Design review of the part built by this model. Coordinates are the model's own, in mm. A direction names the side the tool comes from. Give positions to 0.01 mm unless a question says otherwise; leave off trailing zeros. Write each loop counter-clockwise with the first axis right and the second up, starting at its lowest first coordinate (ties: lowest second). Pieces come first, ordered by that corner, then holes. Notation, with made-up numbers: M 80,17.25 L 126,17.25 A7 cw 126,27.25 Z; hole C 81,53.25 d7. An arc over 180 degrees is marked long. Write each question's results on one line, items separated by ' | '. Start each with the question number.
from build123d import *

# Parameters (mm, degrees)
SKETCH1_W                = 40
SKETCH1_H                = 30
BOSS_EXTRUDE1_DEPTH      = 90
SHELL1_T                 = -4
FILLET1_R                = 5
CUT_EXTRUDE1_DEPTH       = 94.407708461
CUT_EXTRUDE1_DEPTH_BACK  = 94.407708461
CUT_EXTRUDE2_DEPTH       = 94.407708461
CUT_EXTRUDE2_DEPTH_BACK  = 94.407708461
SKETCH3_W                = 17.5
SKETCH3_H                = 40
SKETCH5_W                = 2
SKETCH5_H                = 40
BOSS_EXTRUDE2_DEPTH      = 3
SKETCH6_W                = 2
SKETCH6_H                = 18
BOSS_EXTRUDE3_DEPTH      = 3
SKETCH8_W                = 50
SKETCH8_H                = 50
BOSS_EXTRUDE4_DEPTH      = 18
SKETCH10_W               = 45
SKETCH10_H               = 10
CUT_EXTRUDE4_DEPTH       = 37.5
BOSS_EXTRUDE5_REACH      = 103.502
SKETCH15_W               = 10
SKETCH15_H               = 10
CUT_EXTRUDE8_DEPTH       = 103.988587343
CUT_EXTRUDE8_DEPTH_BACK  = 103.988587343
SKETCH20_R               = 2
SKETCH21_R               = 4
CUT_EXTRUDE9_DEPTH       = 5
SKETCH23_W               = 2
SKETCH23_H               = 15
CUT_EXTRUDE10_DEPTH      = 10
CUT_EXTRUDE11_START      = -10
SKETCH24_R               = 1.5
CUT_EXTRUDE11_DEPTH      = 116.031657717
CUT_EXTRUDE12_DEPTH      = 99.140965569
CUT_EXTRUDE12_DEPTH_BACK = 99.140965569
SKETCH27_W               = 50
SKETCH27_H               = 25
SKETCH29_W               = 50
SKETCH29_H               = 2
CUT_EXTRUDE13_DEPTH      = 2
SKETCH30_W               = 50
SKETCH30_H               = 2
CUT_EXTRUDE14_DEPTH      = 2
CUT_EXTRUDE15_DEPTH      = 99.140965569
CUT_EXTRUDE15_DEPTH_BACK = 99.140965569
SKETCH31_R               = 2
SKETCH33_R               = 4
CUT_EXTRUDE16_DEPTH      = 15


with BuildPart() as part:
    # Sketch1 → Boss-Extrude1 (new body)
    with BuildSketch(Plane(origin=(0, 0, 0), x_dir=(1, 0, 0), z_dir=(0, 1, 0))):
        Rectangle(SKETCH1_W, SKETCH1_H)
    extrude(amount=BOSS_EXTRUDE1_DEPTH)

    # Shell1
    shell1_openings = [part.faces().sort_by_distance(p)[0] for p in [
        (0, 90, 0),
        (0, 0, 0),
    ]]
    offset(amount=SHELL1_T, openings=shell1_openings, kind=Kind.INTERSECTION)

    # Fillet1
    fillet1_edges = [part.edges().sort_by_distance(p)[0] for p in [
        (20, 45, 15),
        (-20, 45, 15),
        (-20, 45, -15),
        (20, 45, -15),
    ]]
    fillet(fillet1_edges, radius=FILLET1_R)

    # Sketch2 → Cut-Extrude1 (cut, two sides: drawn at the far end of the back side and taken through both)
    with BuildSketch(Plane.XY.offset(-CUT_EXTRUDE1_DEPTH_BACK)):
        Polygon((-5.5, 90), (-20, 66), (-20, 90), align=None)
    extrude(amount=CUT_EXTRUDE1_DEPTH + CUT_EXTRUDE1_DEPTH_BACK, mode=Mode.SUBTRACT)

    # Sketch3 → Cut-Extrude2 (cut, two sides: drawn at the far end of the back side and taken through both)
    with BuildSketch(Plane.XY.offset(-CUT_EXTRUDE2_DEPTH_BACK)):
        with Locations((11.25, 70)):
            Rectangle(SKETCH3_W, SKETCH3_H)
    extrude(amount=CUT_EXTRUDE2_DEPTH + CUT_EXTRUDE2_DEPTH_BACK, mode=Mode.SUBTRACT)

    # Sketch5 → Boss-Extrude2 (add)
    with BuildSketch(Plane(origin=(2.5, 0, 0), x_dir=(0, 0, -1), z_dir=(1, 0, 0))):
        with Locations((-13, 70)):
            Rectangle(SKETCH5_W, SKETCH5_H)
    boss_extrude2 = extrude(amount=BOSS_EXTRUDE2_DEPTH)

    # Mirror1: Boss-Extrude2 across plane
    add(boss_extrude2.mirror(Plane.XY))

    # Sketch6 → Boss-Extrude3 (add)
    with BuildSketch(Plane(origin=(-43.86391097, 26.501112878, 0), x_dir=(0, 0, 1), z_dir=(-0.8559155419457906, 0.5171156399255814, 0))):
        with Locations((-13, 65.188262756)):
            Rectangle(SKETCH6_W, SKETCH6_H)
    boss_extrude3 = extrude(amount=BOSS_EXTRUDE3_DEPTH)

    # Mirror2: Boss-Extrude3 across plane
    add(boss_extrude3.mirror(Plane.XY))

    # Sketch8 → Boss-Extrude4 (add)
    with BuildSketch(Plane(origin=(0, 0, 0), x_dir=(1, 0, 0), z_dir=(0, 1, 0))):
        Rectangle(SKETCH8_W, SKETCH8_H)
    extrude(amount=-BOSS_EXTRUDE4_DEPTH)

    # Sketch10 → Cut-Extrude4 (cut)
    with BuildSketch(Plane.ZY.offset(25)):
        with Locations((0, -9)):
            Rectangle(SKETCH10_W, SKETCH10_H)
    extrude(amount=-CUT_EXTRUDE4_DEPTH, mode=Mode.SUBTRACT)

    # Sketch15 → Boss-Extrude5 (add, up to next)
    with BuildSketch(Plane.XY.offset(-11), mode=Mode.PRIVATE) as boss_extrude5_sk1:
        with Locations((-11, 5)):
            Rectangle(SKETCH15_W, SKETCH15_H)
    boss_extrude5_tool1 = extrude(boss_extrude5_sk1.sketch, amount=BOSS_EXTRUDE5_REACH, mode=Mode.PRIVATE) - part.part
    add(boss_extrude5_tool1.solids().sort_by_distance((-11, 5, -11))[0])

    # Sketch20 → Cut-Extrude8 (cut, two sides: drawn at the far end of the back side and taken through both)
    with BuildSketch(Plane(origin=(0, 0, -15), x_dir=(-1, 0, 0), z_dir=(0, 0, -1)).offset(-CUT_EXTRUDE8_DEPTH_BACK)):
        with Locations((11, 5)):
            Circle(SKETCH20_R)
    extrude(amount=CUT_EXTRUDE8_DEPTH + CUT_EXTRUDE8_DEPTH_BACK, mode=Mode.SUBTRACT)

    # Sketch21 → Cut-Extrude9 (cut)
    with BuildSketch(Plane(origin=(0, 0, -15), x_dir=(-1, 0, 0), z_dir=(0, 0, -1))):
        with Locations((11, 5)):
            Circle(SKETCH21_R)
    cut_extrude9 = extrude(amount=-CUT_EXTRUDE9_DEPTH, mode=Mode.SUBTRACT)

    # Mirror3: Cut-Extrude9 across plane
    add(cut_extrude9.mirror(Plane.XY), mode=Mode.SUBTRACT)

    # Sketch23 → Cut-Extrude10 (cut)
    with BuildSketch(Plane(origin=(0, 50, 0), x_dir=(1, 0, 0), z_dir=(0, 1, 0))):
        with Locations((17.949489743, 0)):
            Rectangle(SKETCH23_W, SKETCH23_H)
    extrude(amount=-CUT_EXTRUDE10_DEPTH, mode=Mode.SUBTRACT)

    # Sketch24 → Cut-Extrude11 (cut)
    with BuildSketch(Plane(origin=(20, 0, 0), x_dir=(0, 0, -1), z_dir=(1, 0, 0)).offset(CUT_EXTRUDE11_START)):
        with Locations(Location((-5, 46, 0), (0, 0, 180))):
            Circle(SKETCH24_R)
    cut_extrude11 = extrude(amount=CUT_EXTRUDE11_DEPTH, mode=Mode.SUBTRACT)

    # Mirror4: Cut-Extrude11 across plane
    add(cut_extrude11.mirror(Plane.XY), mode=Mode.SUBTRACT)

    # Sketch27 → Cut-Extrude12 (cut, two sides: drawn at the far end of the back side and taken through both)
    with BuildSketch(Plane(origin=(0, 0, 0), x_dir=(1, 0, 0), z_dir=(0, 1, 0)).offset(-CUT_EXTRUDE12_DEPTH_BACK)):
        with Locations((0, -12.5)):
            Rectangle(SKETCH27_W, SKETCH27_H)
    extrude(amount=CUT_EXTRUDE12_DEPTH + CUT_EXTRUDE12_DEPTH_BACK, mode=Mode.SUBTRACT)

    # Sketch29 → Cut-Extrude13 (cut)
    with BuildSketch(Plane.XY):
        with Locations((0, -2)):
            Rectangle(SKETCH29_W, SKETCH29_H)
    extrude(amount=-CUT_EXTRUDE13_DEPTH, mode=Mode.SUBTRACT)

    # Sketch30 → Cut-Extrude14 (cut)
    with BuildSketch(Plane.XY):
        with Locations((0, -16)):
            Rectangle(SKETCH30_W, SKETCH30_H)
    extrude(amount=-CUT_EXTRUDE14_DEPTH, mode=Mode.SUBTRACT)

    # Sketch31 → Cut-Extrude15 (cut, two sides: drawn at the far end of the back side and taken through both)
    with BuildSketch(Plane.XY.offset(-CUT_EXTRUDE15_DEPTH_BACK)):
        with Locations((17, -9)):
            Circle(SKETCH31_R)
    extrude(amount=CUT_EXTRUDE15_DEPTH + CUT_EXTRUDE15_DEPTH_BACK, mode=Mode.SUBTRACT)

    # Sketch33 → Cut-Extrude16 (cut)
    with BuildSketch(Plane(origin=(0, 0, -25), x_dir=(-1, 0, 0), z_dir=(0, 0, -1))):
        with Locations((-17, -9)):
            Circle(SKETCH33_R)
    extrude(amount=-CUT_EXTRUDE16_DEPTH, mode=Mode.SUBTRACT)


solid = part.part
Q1. We need section A-A on z = -5. Count the separate pieces of the cut face and the enclosed holes in it, and give its area (3 significant figures).
Q2. The part is to be moulded in two halves that separate along Y. For faces 1 (the flat face through (-6, 5, -6)), 2 (the cylindrical face through (19.467, 47.464, -4.675)), 3 (the flat face through (0, 90, -13)), 4 (the flat face through (12.5, -9, -11)), say which applies: pulls with the +Y half, pulls with the -Y half, needs draft (parallel to the pull), parting line crosses it, or undercut.
Q3. We need section B-B on x = -3. Write out the cut boundary in (y, z).
Q4. For faces 5 (the flat face through (-7, -14, -11)), 6 (the cylindrical face through (19, 25, -13)), 7 (the flat face through (20, 25, -5)), 8 (the flat face through (-16, 41, -5)), 9 (the flat face through (0, -16, -2)), list the 3-axis set-ups (+Z, -Z, +X, -X, +Y, -Y) from which the entire face can be reached by the end or side of a thin tool; tool diameter is ignored.
Q5. We need section D-D on z = -21.5. Write out the cut boundary in (x, y), and give its area (3 significant figures).
Q6. We need section C-C on y = 46. Write out the cut boundary in (x, z), and give its area (3 significant figures).
Q7. For pin 1 Ø0.9 at (x, y) = (4, 63.5) entering from -Z; pin 2 Ø4 at (x, y) = (9, 14) entering from +Z; pin 3 Ø2 at (y, z) = (73, -13) entering from +X; pin 4 Ø1.5 at (y, z) = (47, -17) entering from -X (3 decimals), all flat-tipped, find the tip position at first contact; note any pin that passes through.
Q8. Wall thickness on line 1 along Y through (x, z) = (-11, -4.25); line 2 along X through (y, z) = (5, -6); line 3 along Y through (x, z) = (-17.5, -16.5): over which ranges is each line inside the solid? List them lowest first. Write a range as from..to.
Answer sheet:
1) separate pieces: 3 | enclosed holes: 2 | area: 1,050 mm^2
2) face 1: needs draft | face 2: undercut | face 3: pulls with the +Y half | face 4: undercut
3) outline: M -18,-25 L 0,-25 L 0,-15 L 90,-15 L 90,-11 L 0,-11 L 0,0 L -1,0 L -1,-2 L -3,-2 L -3,0 L -4,0 L -4,-22.5 L -14,-22.5 L -14,0 L -15,0 L -15,-2 L -17,-2 L -17,0 L -18,0 Z
4) face 5: +Z, -X | face 6: -Z, +X, +Y | face 7: +Z, -Z, +X, +Y | face 8: +Z, +Y | face 9: +Z, +X, -X
5) outline: M -25,-18 L 25,-18 L 25,0 L -25,0 L -25,-4 L 12.5,-4 L 12.5,-14 L -25,-14 Z; hole C 17,-9 d8 | area: 475 mm^2
6) outline: M -20,-10 A5 ccw -15,-15 L 15,-15 A5 ccw 20,-10 L 20,-6.5 L 18.95,-6.5 L 18.95,-7.5 L 16.95,-7.5 L 16.95,-6.5 L 16,-6.5 L 16,-11 L -16,-11 L -16,0 L -20,0 Z; M 16,-3.5 L 16.95,-3.5 L 16.95,0 L 16,0 Z; M 18.95,-3.5 L 20,-3.5 L 20,0 L 18.95,0 Z | area: 216 mm^2
7) pin 1: z = -14 | pin 2: z = -11 | pin 3: x = 5.5 | pin 4: through
8) line 1: -18..-14, -4..3, 7..10 | line 2: -20..-13, -9..-6, 16..20 | line 3: -18..-14, -4..0
